Can you work these out from the model? Positions are in its coordinate system, mm. Face numbers are marked on the shaded views. A direction names the side the tool comes from. Round coordinates to 2 decimals unless told otherwise and drop trailing zeros. Order: outer loops, then holes, each group sorted by start corner. A loop starts at its lowest first (then second) coordinate and runs counter-clockwise, first axis right, second up.
Q1. For the marked faces 1, 2 and 3, which set-ups out of +Z, -Z, +X, -X, +Y, -Y let a thin tool reach every point of the face, with its end or its side?
Q2. Will these pins go through, and if not, where does the flat tip stop? P1, Ø1.5, axis at x = 4.5, y = 14.5, coming from the +Z side; P2, Ø1.5, axis at x = 3, z = -14.5, coming from the +Y side; P3, Ø3.5, axis at x = 3.175, z = -3.175, coming from the -Y side.
Q3. If I drill on line 1 (Z direction, x = 2.5, y = 13.5); line 2 (Z direction, x = 2.25, y = 14.5); line 3 (Y direction, x = 1.5, z = -17.5), over which ranges is the centre line in solid material (lowest first)?
Q4. If we section it at D-D (z = -17.5): Please give me the cut outline in (x, y).
Q5. If we section it at A-A (x = 1.25): Please give me the cut outline in (y, z), plus the area to 3 significant figures.
Q6. If we section it at B-B (z = -4): Please give me the cut outline in (x, y), plus the area to 3 significant figures.
Q7. If we section it at C-C (y = 10.75): Please give me the cut outline in (x, z) (3 decimals).
from build123d import *

# Parameters (mm, degrees)
BOSS_EXTRUDE1_DEPTH           = 6.35
SKETCH2_W                     = 6.35
SKETCH2_H                     = 6.35
BOSS_EXTRUDE2_DEPTH           = 30.48
SKETCH10_W                    = 6.35
SKETCH10_H                    = 6.1722
BOSS_EXTRUDE3_DEPTH           = 1.016
TAP_DRILL_FOR_6_32_TAP4_D     = 2.7051
TAP_DRILL_FOR_6_32_TAP4_DEPTH = 6.35
TAP_DRILL_FOR_6_32_TAP4_TIP   = 0.81269403
TAP_DRILL_FOR_6_32_TAP3_D     = 2.7051
SKETCH13_W                    = 6.35
SKETCH13_H                    = 30.48
CUT_EXTRUDE1_DEPTH            = 0.0889
SKETCH14_W                    = 6.35
SKETCH14_H                    = 30.48
CUT_EXTRUDE2_DEPTH            = 0.0889
SKETCH15_W                    = 6.35
SKETCH15_H                    = 1.016
CUT_EXTRUDE3_DEPTH            = 0.0889
SKETCH16_W                    = 6.35
SKETCH16_H                    = 1.016
CUT_EXTRUDE4_DEPTH            = 0.0889


with BuildPart() as part:
    # Sketch1 → Boss-Extrude1 (new body)
    with BuildSketch(Plane(origin=(0, 0, 0), x_dir=(0, 0, -1), z_dir=(1, 0, 0))):
        Polygon((0, 0), (0, 25.4), (-2.032, 25.4), (-16.696696837, 0), align=None)
    extrude(amount=BOSS_EXTRUDE1_DEPTH)

    # Sketch2 → Boss-Extrude2 (add)
    with BuildSketch(Plane(origin=(0, 0, 0), x_dir=(-1, 0, 0), z_dir=(0, 0, -1))):
        with Locations((-3.175, 12.7)):
            Rectangle(SKETCH2_W, SKETCH2_H)
    extrude(amount=BOSS_EXTRUDE2_DEPTH)

    # Sketch10 → Boss-Extrude3 (add)
    with BuildSketch(Plane(origin=(0, 7.22988181, 12.522522628), x_dir=(1, 0, 0), z_dir=(0, 0.49999999999999467, 0.8660254037844417))):
        with Locations((3.175, 3.035945256)):
            Rectangle(SKETCH10_W, SKETCH10_H)
    extrude(amount=BOSS_EXTRUDE3_DEPTH)

    # Tap Drill for #6-32 Tap4
    with Locations(Plane(origin=(0, 7.22988181, 12.522522628), x_dir=(1, 0, 0), z_dir=(0, 0.49999999999999467, 0.8660254037844417))):
        with Locations((3.175, 10.821045256)):
            Hole(TAP_DRILL_FOR_6_32_TAP4_D / 2, depth=TAP_DRILL_FOR_6_32_TAP4_DEPTH)
            with Locations((0, 0, -(TAP_DRILL_FOR_6_32_TAP4_DEPTH + TAP_DRILL_FOR_6_32_TAP4_TIP / 2))):  # 118° drill point
                Cone(0, TAP_DRILL_FOR_6_32_TAP4_D / 2, TAP_DRILL_FOR_6_32_TAP4_TIP, mode=Mode.SUBTRACT)

    # Tap Drill for #6-32 Tap3 (through all)
    with Locations(Plane(origin=(0, 15.875, 0), x_dir=(1, 0, 0), z_dir=(0, 1, 0))):
        with Locations((3.175, 3.175), (3.175, 27.559)):
            Hole(TAP_DRILL_FOR_6_32_TAP3_D / 2)

    # Sketch13 → Cut-Extrude1 (cut)
    with BuildSketch(Plane(origin=(0, 15.875, 0), x_dir=(1, 0, 0), z_dir=(0, 1, 0))):
        with Locations((3.175, 15.24)):
            Rectangle(SKETCH13_W, SKETCH13_H)
    extrude(amount=-CUT_EXTRUDE1_DEPTH, mode=Mode.SUBTRACT)

    # Sketch14 → Cut-Extrude2 (cut)
    with BuildSketch(Plane.XZ.offset(-9.525)):
        with Locations((3.175, -15.24)):
            Rectangle(SKETCH14_W, SKETCH14_H)
    extrude(amount=-CUT_EXTRUDE2_DEPTH, mode=Mode.SUBTRACT)

    # Sketch15 → Cut-Extrude3 (cut)
    with BuildSketch(Plane(origin=(0, 5.301846715, -3.061022628), x_dir=(1, 0, 0), z_dir=(0, 0.8660254037844417, -0.49999999999999467))):
        with Locations((3.175, -14.96776362)):
            Rectangle(SKETCH15_W, SKETCH15_H)
    extrude(amount=-CUT_EXTRUDE3_DEPTH, mode=Mode.SUBTRACT)

    # Sketch16 → Cut-Extrude4 (cut)
    with BuildSketch(Plane(origin=(0, -0.043435282, 0.025077372), x_dir=(1, 0, 0), z_dir=(0, -0.8660254037844417, 0.49999999999999467))):
        with Locations((3.175, 14.96776362)):
            Rectangle(SKETCH16_W, SKETCH16_H)
    extrude(amount=-CUT_EXTRUDE4_DEPTH, mode=Mode.SUBTRACT)


solid = part.part
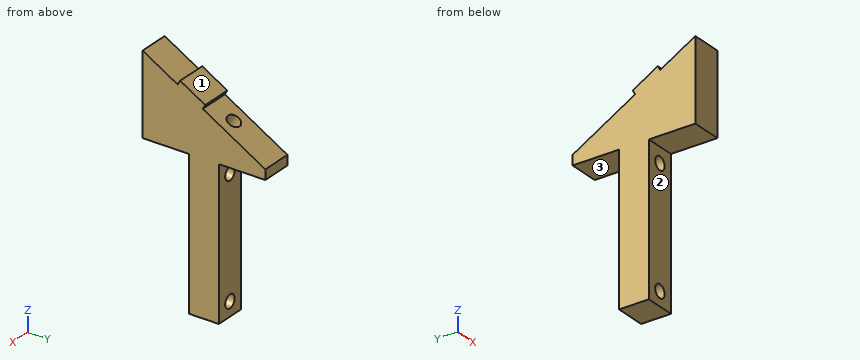
Solution:
1. face 1: +Z, +X, -X, +Y
1. face 2: -Z, +X, -X, -Y
1. face 3: -Z, +X, -X, +Y
2. P1: stops at z = 8.76
2. P2: stops at y = 15.79
2. P3: stops at y = 9.61
3. line 1: z = -30.48 to -28.73, -26.39 to -4.35, -2 to 1.14, 4.08 to 8.9
3. line 2: z = -30.48 to -28.55, -26.57 to -4.16, -2.19 to 1.5, 5.45 to 8.33
3. line 3: y = 9.61 to 15.79
4. outline: (0, 9.61) - (6.35, 9.61) - (6.35, 15.79) - (0, 15.79) - close
5. outline: (0, 0) - (9.61, 0) - (9.61, -30.48) - (15.79, -30.48) - (15.79, 0) - (25.4, 0) - (25.4, 2.03) - (12.45, 9.51) - (12.96, 10.39) - (7.77, 13.38) - (7.26, 12.5) - (0, 16.7) - close
5. area: 432 mm2
6. outline: (0, 9.61) - (2.1, 9.61) - (2.1, 15.79) - (0, 15.79) - close; (4.25, 9.61) - (6.35, 9.61) - (6.35, 15.79) - (4.25, 15.79) - close
6. area: 26.0 mm2
7. outline: (0, -30.48) - (6.35, -30.48) - (6.35, 11.663) - (0, 11.663) - close; hole circle Ø2.705 at (3.175, -27.559); hole circle Ø2.705 at (3.175, -3.175)
